Source: three-view drawing plus pictorial views. Frame: mm from the lowest corner of the part. Round coordinates to 2 decimals unless told otherwise and drop trailing zeros. Write each loop counter-clockwise with the first axis right and the second up, starting at its lowest first coordinate (ties: lowest second). Pieces come first, ordered by that corner, then holes.
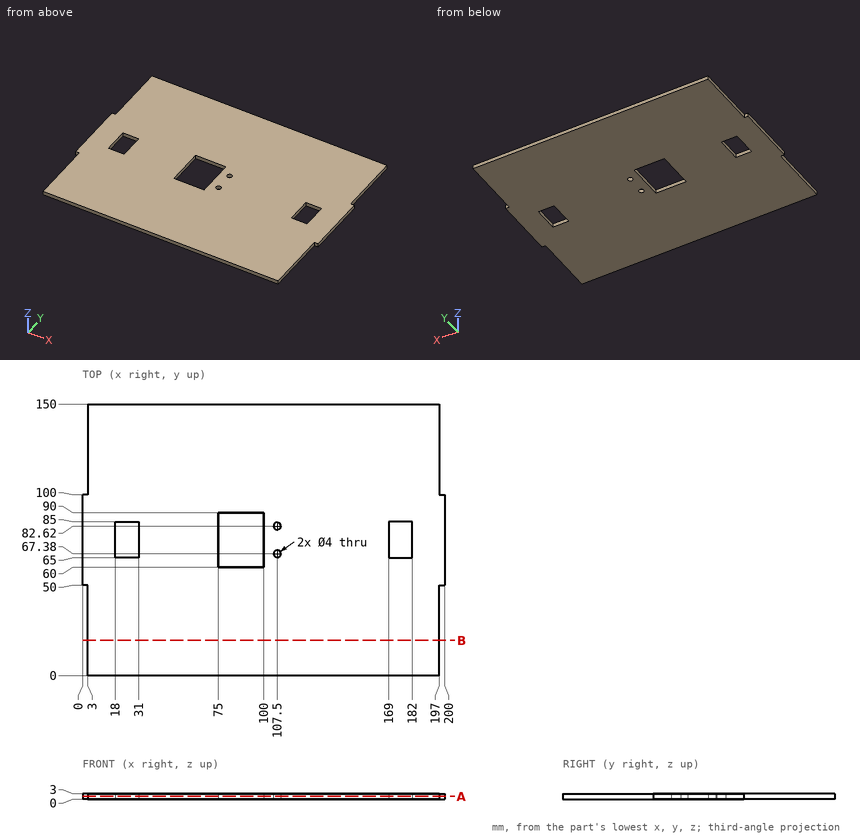
1) Section B-B on y = 19.5. Output: boundary loops of the cut face in (x, z).
2) Section A-A on z = 1.5. Output: boundary loops of the cut face in (x, y), plus the area to 3 significant figures.
3) First-contact query: P1, Ø1, axis at x = 43.5, z = 2.5, coming from the -Y side; P2, Ø1.5, axis at y = 132, z = 2, coming from the +X side; P3, Ø1.5, axis at x = 2, z = 1, coming from the +Y side; P4, Ø0.9, axis at x = 198.5, z = 1, coming from the -Y side. Flat tips, straight axial feed; report the tip coordinate or a pass-through.
4) Line query: probe 1 along Y at (x, z) = (107.5, 2.1); probe 2 along X at (y, z) = (61, 1.3); probe 3 along Y at (x, z) = (18.5, 0.4). Output: solid intervals per line, ascending.
Filled in:
1. outline: (3, 0) - (197, 0) - (197, 3) - (3, 3) - close
2. outline: (0, 50) - (3, 50) - (3, 0) - (197, 0) - (197, 50) - (200, 50) - (200, 100) - (197, 100) - (197, 150) - (3, 150) - (3, 100) - (0, 100) - close; hole (18, 65) - (31, 65) - (31, 85) - (18, 85) - close; hole (75, 60) - (100, 60) - (100, 90) - (75, 90) - close; hole circle Ø4 at (107.5, 67.38); hole circle Ø4 at (107.5, 82.62); hole (169, 65) - (182, 65) - (182, 85) - (169, 85) - close
2. area: 28,100 mm2
3. P1: stops at y = 0
3. P2: stops at x = 197
3. P3: stops at y = 100
3. P4: stops at y = 50
4. probe 1: y = 0 to 65.38, 69.38 to 80.62, 84.62 to 150
4. probe 2: x = 0 to 75, 100 to 200
4. probe 3: y = 0 to 65, 85 to 150
